Check sheet for the modelled part. Datum: model origin and axes. Units: mm. A direction names the side the tool comes from. Round coordinates to 2 decimals unless told otherwise and drop trailing zeros. Order: outer loops, then holes, each group sorted by start corner. A loop starts at its lowest first (then second) coordinate and runs counter-clockwise, first axis right, second up. Notation, with made-up numbers: (25, 82) -> (40, 82) arc R20 ccw to (40, 114) -> close; hole circle Ø8 at (53.5, 62). An arc over 180 degrees is marked (long way). Answer in a Markdown table with one row per item.
from build123d import *

# Parameters (mm, degrees)
BOSS_EXTRUDE2_DEPTH = 5
BOSS_EXTRUDE3_DEPTH = 5
SKETCH3_R           = 0.71884788
CUT_EXTRUDE1_DEPTH  = 5


# Read off the part's stored shape, not the designer's step: Boss-Extrude3
with BuildPart() as part:
    # Sketch1 → Boss-Extrude2 (new body)
    with BuildSketch(Plane.XY):
        with BuildLine():
            Line((-7.366666667, -4.240545038), (-6.5, -3.741657387))
            ThreePointArc((-6.5, -3.741657387), (-7.245688373, -1.936491673), (-7.5, 0))
            ThreePointArc((-7.5, 0), (0, 7.5), (7.5, 0))
            ThreePointArc((7.5, 0), (7.245688373, -1.936491673), (6.5, -3.741657387))
            Line((6.5, -3.741657387), (7.366666667, -4.240545038))
            ThreePointArc((7.366666667, -4.240545038), (8.211780156, -2.194690563), (8.5, 0))
            ThreePointArc((8.5, 0), (0, 8.5), (-8.5, 0))
            ThreePointArc((-8.5, 0), (-8.211780156, -2.194690563), (-7.366666667, -4.240545038))
        make_face()
    extrude(amount=BOSS_EXTRUDE2_DEPTH)

    # Boss-Extrude3 outline → Boss-Extrude3 (add)
    with BuildSketch(Plane.XY):
        with BuildLine():
            Line((-7.924926196, 4.802995865), (-7.365135024, 4.243204694))
            ThreePointArc((-7.365135024, 4.243204694), (-5.790125857, 6.222896638), (-3.702233025, 7.651370506))
            Line((-3.702233025, 7.651370506), (-4.38939229, 8.338529771))
            Line((-4.38939229, 8.338529771), (-7.924926196, 4.802995865))
        make_face()
    extrude(amount=BOSS_EXTRUDE3_DEPTH)

    # Sketch3 → Cut-Extrude1 (cut)
    with BuildSketch(Plane(origin=(-6.363961031, 6.363961031, 0), x_dir=(0, 0, 1), z_dir=(-0.7071067811865476, 0.7071067811865476, 0))):
        with Locations(Location((2.5, 0.292461893, 0), (0, 0, 270))):
            Circle(SKETCH3_R)
    extrude(amount=-CUT_EXTRUDE1_DEPTH, mode=Mode.SUBTRACT)


solid = part.part
Item 1: Cross-section at C-C (x = -7). Record the boundary of the cut face in (y, z), and give its area (3 significant figures).
Result sheet:
| item | result |
|---|---|
| outline | (-4.03, 0) -> (-2.69, 0) -> (-2.69, 5) -> (-4.03, 5) -> close; (2.69, 0) -> (5.73, 0) -> (5.73, 5) -> (2.69, 5) -> close |
| area | 21.9 mm^2 |
Item 2: Cross-section at A-A (y = 3). Record the boundary of the cut face in (x, z), and give its area (3 significant figures).
Result sheet:
| item | result |
|---|---|
| outline | (-7.95, 0) -> (-6.87, 0) -> (-6.87, 5) -> (-7.95, 5) -> close; (6.87, 0) -> (7.95, 0) -> (7.95, 5) -> (6.87, 5) -> close |
| area | 10.8 mm^2 |
Item 3: Set-up check for faces 4 (the flat face through (-6.13, 6.6, 1.35)), 5 (the flat face through (6.93, -3.99, 2.46)): record each of +Z, -Z, +X, -X, +Y, -Y from which the full face is reachable in a straight line by a thin tool's end or side.
Result sheet:
| item | result |
|---|---|
| face 4 | +Z, -Z, -X, +Y |
| face 5 | +Z, -Z, -Y |
Item 4: Cross-section at B-B (z = 4.2). Record the boundary of the cut face in (x, y), and give its area (3 significant figures).
Result sheet:
| item | result |
|---|---|
| outline | (-7.92, 4.8) -> (-7.37, 4.24) arc R8.5 ccw to (-7.37, -4.24) -> (-6.5, -3.74) arc R7.5 cw (long way) to (6.5, -3.74) -> (7.37, -4.24) arc R8.5 ccw to (-3.7, 7.65) -> (-4.39, 8.34) -> close |
| area | 36.6 mm^2 |
Item 5: Mould release check, pull along Z, two halves, no side actions. Record for faces 1 (the cylindrical face through (-6.08, 5.554, 2.225)), 2 (the flat face through (-6.939, -3.995, 2.465)), 3 (the flat face through (-2.6, 7.4, 5)): pulls with the +Z half, pulls with the -Z half, needs draft (parallel to the pull), parting line crosses it, or undercut.
Result sheet:
| item | result |
|---|---|
| face 1 | undercut |
| face 2 | needs draft |
| face 3 | pulls with the +Z half |
Item 6: Cross-section at D-D (x = 0). Record the boundary of the cut face in (y, z).
Result sheet:
| item | result |
|---|---|
| outline | (7.5, 0) -> (8.5, 0) -> (8.5, 5) -> (7.5, 5) -> close |
Item 7: Scan lines: line 1 (X direction, y = -3, z = 4.75); line 2 (X direction, y = -1.75, z = 1.4); line 3 (Y direction, x = -5.5, z = 0.55). Record each from-to range of solid material in increasing order. Write a range as [from, to].
Result sheet:
| item | result |
|---|---|
| line 1 | x = [-7.95, -6.87], [6.87, 7.95] |
| line 2 | x = [-8.32, -7.29], [7.29, 8.32] |
| line 3 | y = [5.1, 7.23] |
Item 8: Depth check by flat-ended pin: P1, Ø1, axis at x = -5, y = -1.5, coming from the -Z side; P2, Ø2, axis at y = 3, z = 1.5, coming from the -X side; P3, Ø1.5, axis at x = 2, z = 0.5, coming from the -Y side. Enter the tip coordinate at first touch or a pass-through.
Result sheet:
| item | result |
|---|---|
| P1 | passes through |
| P2 | stops at x = -8.26 |
| P3 | stops at y = 6.98 |
